Input: part model. Units: mm. Frame: model coordinates. Face numbers are marked on the shaded views. A direction names the side the tool comes from. Coordinates: 2 decimals unless noted, no trailing zeros. Loops run counter-clockwise (first coordinate to the right, second up) from the corner with the lowest first, then second, coordinate; pieces in that order, holes last. Notation, with made-up numbers: (57.5, 8.25) - (99.5, 8.25) arc R20 ccw to (99.5, 21.25) - close; hole circle Ø6 at (17.5, 20.5). An arc over 180 degrees is marked (long way). Use a Markdown table: item, result. Add a question column.
1. Contact query for flat-ended pins moving along their axis: P1, Ø3, axis at x = -23, z = 2.5, coming from the -Y side; P2, Ø1, axis at x = -6.5, y = -0.5, coming from the -Z side; P3, Ø1.5, axis at x = -7.5, y = -1.5, coming from the +Z side. Output: stop coordinate, or through.
2. Access query for the marked faces 1 and 2. Directions: +Z, -Z, +X, -X, +Y, -Y. A direction counts if a zero-diameter tool reaches every point of the face in a straight line with its end or side. Return the directions, or none.
3. Ray query, L1, parallel to X at y = 0.25, z = 3.25; L2, parallel to X at y = -0.5, z = 0; L3, parallel to Z at x = -11.5, y = -0.25. Return the intervals inside material, ascending. Write a range as [from, to].
4. Section query B-B on z = -2.5. Return the cut outline in (x, y).
5. Section query A-A on x = -24. Return the cut outline in (y, z), then the cut area to 3 significant figures.
```python
from build123d import *

# Parameters (mm, degrees)
SKETCH2_R           = 2
BOSS_EXTRUDE1_DEPTH = 35
CHAMFER1_SIZE       = 0.3
SKETCH6_W           = 2.8
SKETCH6_H           = 3.5
CUT_EXTRUDE1_DEPTH  = 1.6
SKETCH8_R           = 1.493375673
CUT_EXTRUDE2_DEPTH  = 1
CUT_EXTRUDE2_TAPER  = 45


with BuildPart() as part:
    # Sketch2 → Boss-Extrude1 (new body)
    with BuildSketch(Plane(origin=(0, 0, 0), x_dir=(0, 0, -1), z_dir=(1, 0, 0))):
        Circle(SKETCH2_R)
    extrude(amount=-BOSS_EXTRUDE1_DEPTH)

    # Chamfer1
    chamfer1_edges = [part.edges().sort_by_distance(p)[0] for p in [
        (0, 0, 2),
    ]]
    chamfer(chamfer1_edges, length=CHAMFER1_SIZE)

    # Sketch6 → Revolve1 (revolve)
    with BuildSketch(Plane.XY):
        with Locations((-36.4, 1.75)):
            Rectangle(SKETCH6_W, SKETCH6_H)
    revolve(axis=Axis((-35, 0, 0), (1, 0, 0)))

    # Sketch7 → Cut-Extrude1 (cut)
    with BuildSketch(Plane.ZY.offset(37.8)):
        Polygon((0, 1.443375673), (-1.25, 0.721687836), (-1.25, -0.721687836), (0, -1.443375673), (1.25, -0.721687836), (1.25, 0.721687836), align=None)
    extrude(amount=-CUT_EXTRUDE1_DEPTH, mode=Mode.SUBTRACT)

    # Sketch8 → Cut-Extrude2 (cut)
    with BuildSketch(Plane.ZY.offset(37.8)):
        Circle(SKETCH8_R)
    extrude(amount=-CUT_EXTRUDE2_DEPTH, taper=CUT_EXTRUDE2_TAPER, mode=Mode.SUBTRACT)


solid = part.part
```
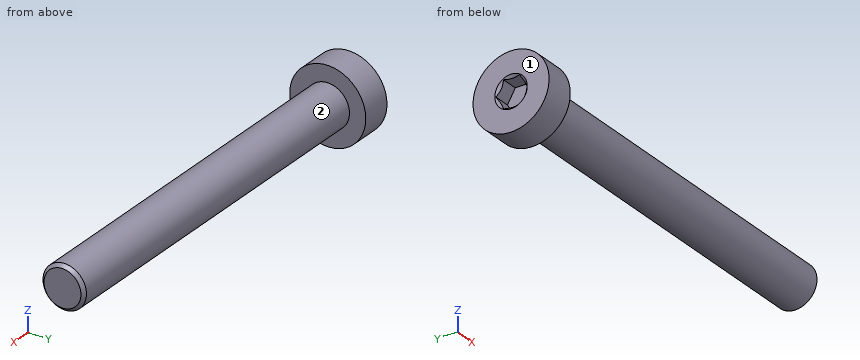
Resolved:
| question | item | result |
|---|---|---|
| 1 | P1 | y = -1.73 |
| 1 | P2 | z = -2 |
| 1 | P3 | z = 1.85 |
| 2 | face 1 | +Z, -Z, -X, +Y, -Y |
| 2 | face 2 | +X |
| 3 | L1 | [-37.8, -35] |
| 3 | L2 | [-36.2, 0] |
| 3 | L3 | [-1.98, 1.98] |
| 4 | outline | (-37.8, -2.45) - (-35, -2.45) - (-35, 2.45) - (-37.8, 2.45) - close |
| 5 | outline | circle Ø4 at (0, 0) |
| 5 | area | 12.6 mm² |
